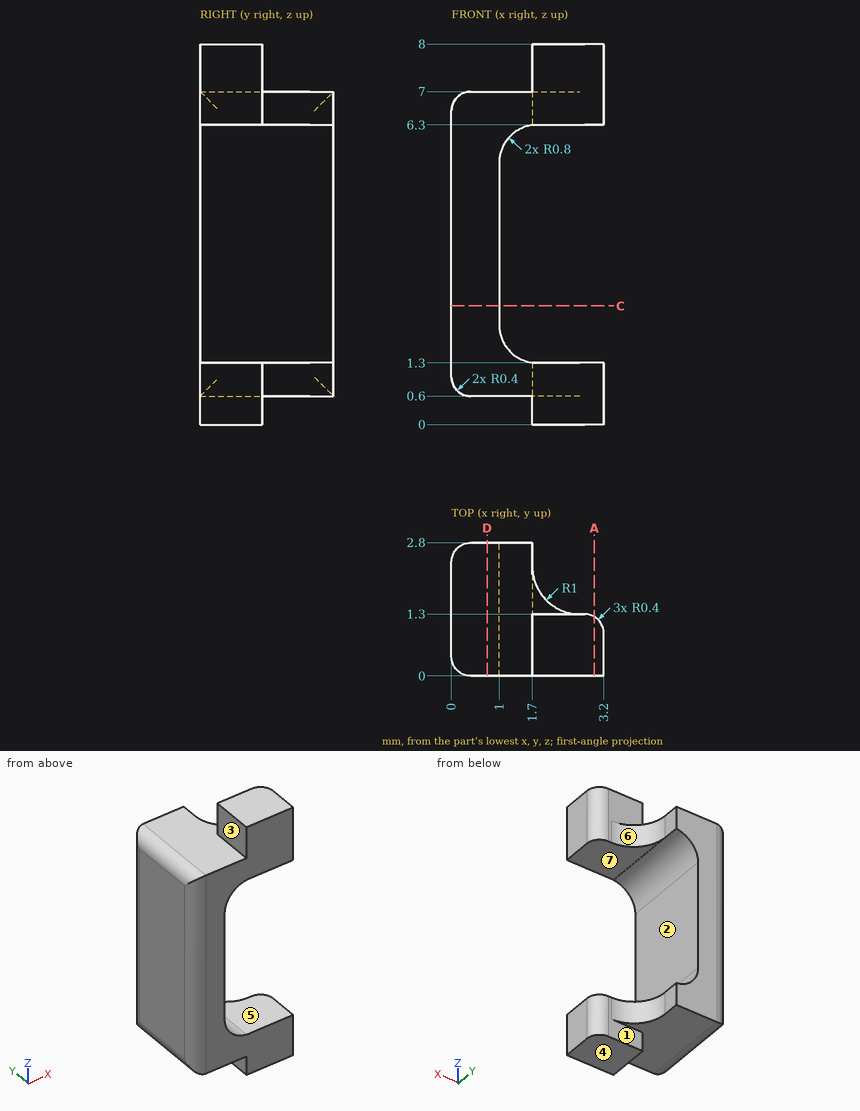
Could you check a few things on this drawing? It's one solid part, dimensions in mm from its lowest x, y, z. A direction names the side the tool comes from. Coordinates: 2 decimals unless noted, no trailing zeros. Loops run counter-clockwise (first coordinate to the right, second up) from the corner with the lowest first, then second, coordinate; pieces in that order, holes last.
1. Imagine slicing it at D-D (x = 0.75). Please give me the cut outline in (y, z), and give its area (3 significant figures).
2. For the marked faces 1, 2 and 3, which set-ups out of +Z, -Z, +X, -X, +Y, -Y let a thin tool reach every point of the face, with its end or its side?
3. For P1, Ø0.8, axis at y = 0.5, z = 7.5, coming from the -X side; P2, Ø0.8, axis at y = 1.5, z = 1, coming from the +X side; P3, Ø0.5, axis at y = 1, z = 0.5, coming from the -X side, each with a flat end and sliding along its axis, tell me the tip position at first contact or that it passes through.
4. I need wall thicknesses on L1, parallel to Z at x = 3.05, y = 1.15; L2, parallel to X at y = 0.1, z = 7.5; L3, parallel to Z at x = 0.45, y = 1.65. Which ranges of each line are inside material? Lowest first, please.
5. Imagine slicing it at A-A (x = 3). Please give me the cut outline in (y, z).
6. Imagine slicing it at C-C (z = 2.5). Please give me the cut outline in (x, y), and give its area (3 significant figures).
7. We'd pull the mould along Z, two halves only. Please class the marked faces 4, 5, 6 and 7: released by +Z, released by -Z, zero draft, split by the parting line, or undercut.
Computed values:
1. outline: (0, 0.6) - (2.8, 0.6) - (2.8, 7) - (0, 7) - close
1. area: 17.9 mm2
2. face 1: -Z, +X, +Y
2. face 2: +X, +Y, -Y
2. face 3: +Z, -X, +Y, -Y
3. P1: stops at x = 1.7
3. P2: stops at x = 3.15
3. P3: stops at x = 0.09
4. L1: z = 0 to 1.3, 6.3 to 8
4. L2: x = 1.7 to 3.2
4. L3: z = 0.6 to 7
5. outline: (0, 0) - (1.25, 0) - (1.25, 1.3) - (0, 1.3) - close; (0, 6.3) - (1.25, 6.3) - (1.25, 8) - (0, 8) - close
6. outline: (0, 0.4) arc R0.4 ccw to (0.4, 0) - (1, 0) - (1, 2.8) - (0.4, 2.8) arc R0.4 ccw to (0, 2.4) - close
6. area: 2.73 mm2
7. face 4: released by -Z
7. face 5: undercut
7. face 6: zero draft
7. face 7: undercut
